Geometry check sheet. Reference: the model listing, model coordinates, mm. A direction names the side the tool comes from. Round coordinates to 2 decimals unless told otherwise and drop trailing zeros. Write each loop counter-clockwise with the first axis right and the second up, starting at its lowest first coordinate (ties: lowest second). Pieces come first, ordered by that corner, then holes. Notation, with made-up numbers: M 17.25,36.5 L 59.25,36.5 A6 cw 59.25,41.5 Z; hole C 72.5,16.25 d3. An arc over 180 degrees is marked long. Use a Markdown table: item, result.
Autodesk Inventor part; units mm, degrees
ref_plane "YZ Plane" through (0, 0, 0) normal (1, 0, 0) x (0, 1, 0)
ref_plane "XZ Plane" through (0, 0, 0) normal (0, 1, 0) x (-1, 0, 0)
ref_plane "XY Plane" through (0, 0, 0) normal (0, 0, 1) x (1, 0, 0)
sketch "Sketch1" plane through (0, 0, 0) normal (0, 0, 1) x (1, 0, 0)
  line L0 (0, 0) -> (50.8, 0)
  line L1 (50.8, 0) -> (50.8, 50.8)
  line L2 (50.8, 50.8) -> (47.625, 50.8)
  line L3 (44.45, 47.625) -> (44.45, 12.7)
  line L4 (38.1, 6.35) -> (3.175, 6.35)
  line L5 (0, 3.175) -> (0, 0)
  arc A0 (3.175, 6.35) -> (0, 3.175) centre (3.175, 3.175) ccw
  arc A1 (47.625, 50.8) -> (44.45, 47.625) centre (47.625, 47.625) ccw
  arc A2 (38.1, 6.35) -> (44.45, 12.7) centre (38.1, 12.7) ccw
  dimension "d0" = 50.8
  dimension "d1" = 6.35
  dimension "d2" = 3.175
  dimension "d3" = 6.35
extrude "Extrusion1" add sketch "Sketch1" along normal blind 190.5
sketch "Sketch2" plane through (0, 0, 0) normal (0, -1, 0) x (1, 0, 0)
  line L0 (0, 0) -> (50.8, 0)
  line L1 (0, 190.5) -> (50.8, 190.5)
  line L2 (0, 0) -> (0, 190.5)
  point P0 (12.7, 177.8)
  point P1 (31.75, 177.8)
  point P2 (12.7, 12.7)
  point P3 (31.75, 12.7)
  dimension "d6" = 19.05
  dimension "d7" = 12.7
  dimension "d8" = 12.7
  dimension "d9" = 12.7
hole "Hole1" at (12.7, 0, 177.8) at (31.75, 0, 177.8) at (12.7, 0, 12.7) at (31.75, 0, 12.7) direction (0, 1, 0) diameter 6.35 end through all
sketch "Sketch3" plane through (50.8, 0, 0) normal (1, 0, 0) x (0, 0, -1)
  line L0 (0, 0) -> (0, 50.8)
  line L1 (0, 50.8) -> (-190.5, 50.8)
  line L2 (-190.5, 0) -> (-190.5, 50.8)
  point P0 (-177.8, 19.05)
  point P1 (-177.8, 38.1)
  point P2 (-12.7, 19.05)
  point P3 (-12.7, 38.1)
  dimension "d17" = 19.05
  dimension "d18" = 12.7
  dimension "d19" = 12.7
  dimension "d20" = 12.7
hole "Hole2" at (50.8, 19.05, 177.8) at (50.8, 38.1, 177.8) at (50.8, 19.05, 12.7) at (50.8, 38.1, 12.7) direction (-1, 0, 0) diameter 6.35 end through all
properties part number "Right Angle" material "Aluminum 6061"
Item 1: Cross-section at D-D, the plane z = 158. Record the cut outline in (x, y) (3 decimals).
Outcome:
| item | result |
|---|---|
| outline | M 0,0 L 50.8,0 L 50.8,50.8 L 47.625,50.8 A3.175 ccw 44.45,47.625 L 44.45,12.7 A6.35 cw 38.1,6.35 L 3.175,6.35 A3.175 ccw 0,3.175 Z |
Item 2: Go/stop test with flat-tipped pins: pin 1 (3 mm diameter, centred on y = 11.5, z = 115.5, fed in from -X); pin 2 (10 mm diameter, centred on x = 36.5, y = 14.5, fed in from +Z); pin 3 (10.5 mm diameter, centred on y = 29.5, z = 118, fed in from -X); pin 4 (8.5 mm diameter, centred on x = 12.7, z = 12.7, fed in from +Y). Record where each tip stops, or that it passes through.
Outcome:
| item | result |
|---|---|
| pin 1 | stops at x = 43.85 |
| pin 2 | passes through |
| pin 3 | stops at x = 44.45 |
| pin 4 | stops at y = 6.35 |
Item 3: Access from +Z, -Z, +X, -X, +Y, -Y to the whole of each face (thin tool, end or side, straight path). Record for faces 1 (the face through (47.581, 35.954, 180.14)), 2 (the face through (21, 6.35, 94)).
Outcome:
| item | result |
|---|---|
| face 1 | +X, -X |
| face 2 | +Z, -Z, -X, +Y |
Item 4: Cross-section at C-C, the plane x = 12.7. Record the cut outline in (y, z) (3 decimals).
Outcome:
| item | result |
|---|---|
| outline | M 0,0 L 6.35,0 L 6.35,9.525 L 0,9.525 Z; M 0,15.875 L 6.35,15.875 L 6.35,174.625 L 0,174.625 Z; M 0,180.975 L 6.35,180.975 L 6.35,190.5 L 0,190.5 Z |
Item 5: Cross-section at B-B, the plane z = 177.8. Record the cut outline in (x, y) (3 decimals), and give its area (3 significant figures).
Outcome:
| item | result |
|---|---|
| outline | M 0,0 L 9.525,0 L 9.525,6.35 L 3.175,6.35 A3.175 ccw 0,3.175 Z; M 15.875,0 L 28.575,0 L 28.575,6.35 L 15.875,6.35 Z; M 34.925,0 L 50.8,0 L 50.8,15.875 L 44.45,15.875 L 44.45,12.7 A6.35 cw 38.1,6.35 L 34.925,6.35 Z; M 44.45,22.225 L 50.8,22.225 L 50.8,34.925 L 44.45,34.925 Z; M 44.45,41.275 L 50.8,41.275 L 50.8,50.8 L 47.625,50.8 A3.175 ccw 44.45,47.625 Z |
| area | 448 mm2 |
Item 6: Cross-section at A-A, the plane y = 38.1. Record the cut outline in (x, z) (3 decimals), and give its area (3 significant figures).
Outcome:
| item | result |
|---|---|
| outline | M 44.45,0 L 50.8,0 L 50.8,9.525 L 44.45,9.525 Z; M 44.45,15.875 L 50.8,15.875 L 50.8,174.625 L 44.45,174.625 Z; M 44.45,180.975 L 50.8,180.975 L 50.8,190.5 L 44.45,190.5 Z |
| area | 1,130 mm2 |
Item 7: Mould release check, pull along Z, two halves, no side actions. Record for faces 3 (the face through (37, 5, 0)), 4 (the face through (45.36, 49.85, 93.92)), 5 (the face through (33.68, 3.22, 180.32)): +Z half, -Z half, draft (parallel to the pull), parting line (faces both ways), or undercut.
Outcome:
| item | result |
|---|---|
| face 3 | -Z half |
| face 4 | draft |
| face 5 | undercut |
Item 8: Material ranges on line 1 along Z through (x, y) = (48, 19.05) (3 decimals); line 2 along X through (y, z) = (5.25, 177.8) (3 decimals); line 3 along Y through (x, z) = (49, 177), recorded low to high. Write a range as from..to.
Outcome:
| item | result |
|---|---|
| line 1 | z = 0..9.525, 15.875..174.625, 180.975..190.5 |
| line 2 | x = 0.772..9.525, 15.875..28.575, 34.925..50.8 |
| line 3 | y = 0..15.98, 22.12..35.03, 41.17..50.8 |
